Verification items for this drawing (mm, ordinates from the low corner). Round coordinates to 2 decimals unless told otherwise and drop trailing zeros. Order: outer loops, then holes, each group sorted by start corner. A loop starts at its lowest first (then second) coordinate and runs counter-clockwise, first axis right, second up. Notation, with made-up numbers: M 47,48 L 66,48 A18 cw 66,70 Z; hole C 66.25,48.25 d5. An arc over 180 degrees is marked long. Use CSV: the item, a comma, the result in double quotes. Start each with the question number.
Q1. Sectioned sample at D-D (z = 3.3). Enter the section's corners in (x, y), and give its area (3 significant figures).
Q2. Sectioned sample at B-B (x = 15). Enter the section's corners in (y, z), and give its area (3 significant figures).
Q3. Sectioned sample at C-C (y = 45). Enter the section's corners in (x, z), and give its area (3 significant figures).
Q4. Scan lines: line 1 (Y direction, x = 85, z = 3.55); line 2 (X direction, y = 41, z = 2.1); line 3 (Y direction, x = 87, z = 0.5). Record each from-to range of solid material in increasing order.
Q5. Sectioned sample at A-A (y = 24). Enter the section's corners in (x, z).
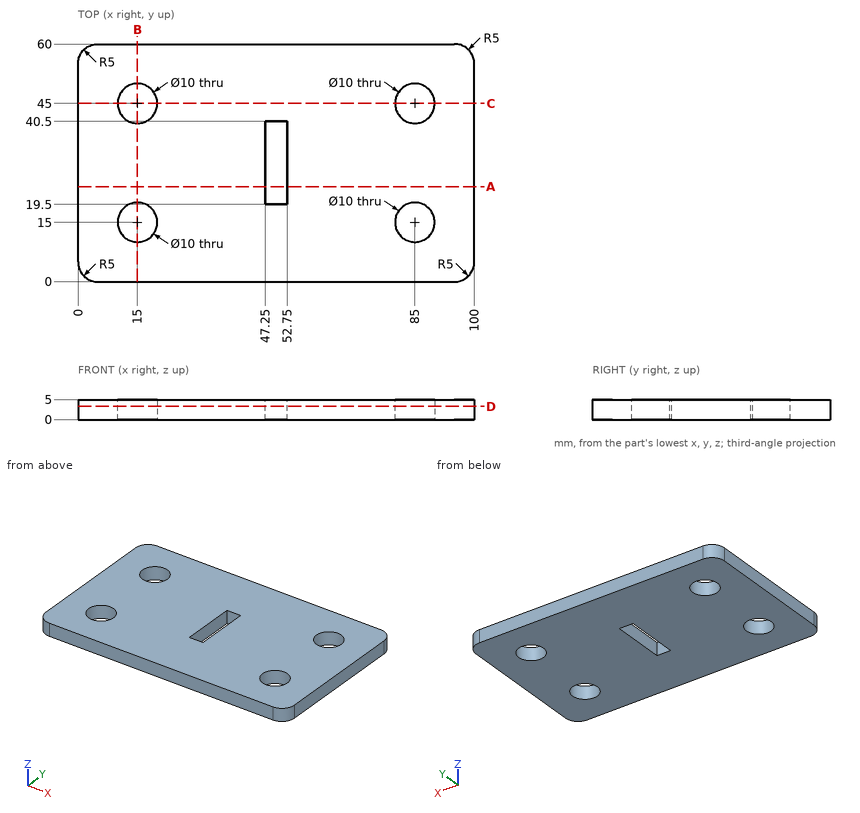
Verdict:
1,outline,"M 0,5 A5 ccw 5,0 L 95,0 A5 ccw 100,5 L 100,55 A5 ccw 95,60 L 5,60 A5 ccw 0,55 Z; hole C 15,15 d10; hole C 15,45 d10; hole M 47.25,19.5 L 52.75,19.5 L 52.75,40.5 L 47.25,40.5 Z; hole C 85,15 d10; hole C 85,45 d10"
1,area,"5,550 mm²"
2,outline,"M 0,0 L 10,0 L 10,5 L 0,5 Z; M 20,0 L 40,0 L 40,5 L 20,5 Z; M 50,0 L 60,0 L 60,5 L 50,5 Z"
2,area,"200 mm²"
3,outline,"M 0,0 L 10,0 L 10,5 L 0,5 Z; M 20,0 L 80,0 L 80,5 L 20,5 Z; M 90,0 L 100,0 L 100,5 L 90,5 Z"
3,area,"400 mm²"
4,line 1,"y = 0 to 10, 20 to 40, 50 to 60"
4,line 2,"x = 0 to 12, 18 to 82, 88 to 100"
4,line 3,"y = 0 to 10.42, 19.58 to 40.42, 49.58 to 60"
5,outline,"M 0,0 L 47.25,0 L 47.25,5 L 0,5 Z; M 52.75,0 L 100,0 L 100,5 L 52.75,5 Z"
